```python
from build123d import *

# Parameters (mm, degrees)
BOSS_EXTRUDE1_DEPTH = 457.2
FILLET1_R           = 152.4


with BuildPart() as part:
    # Sketch1 → Boss-Extrude1 (new body)
    with BuildSketch(Plane(origin=(0, 0, 0), x_dir=(0, 0, -1), z_dir=(1, 0, 0))):
        with BuildLine():
            Line((711.548200753, -160.15002575), (669.063267675, -98.166541557))
            Line((669.063267675, -98.166541557), (-541.133997798, 73.322803393))
            Line((-541.133997798, 73.322803393), (-553.825031188, -16.23759413))
            Line((-553.825031188, -16.23759413), (-581.492567074, -11.395775351))
            Line((-581.492567074, -11.395775351), (-581.492567074, 28.611066701))
            Line((-581.492567074, 28.611066701), (-693.769833475, 31.192153284))
            Line((-693.769833475, 31.192153284), (-711.548200753, -33.910775567))
            Line((-711.548200753, -33.910775567), (-671.038221505, -241.199727441))
            Line((-671.038221505, -241.199727441), (-601.675855782, -250.529122735))
            add(Edge.make_bspline(
                [(-601.675855782, -250.529122735), (-541.133997798, -117.43304901), (-401.043539171, -75.545762029)],
                knots=[0, 0, 0, 1, 1, 1], degree=2, weights=[1, 2.246019703, 1]))
            Line((-401.043539171, -75.545762029), (-324.808759835, -85.222901727))
            Line((-324.808759835, -85.222901727), (-338.797926094, -195.427056695))
            Line((-338.797926094, -195.427056695), (-67.759534981, -212.336640741))
            Line((-67.759534981, -212.336640741), (412.240396354, -324.981912238))
            Line((412.240396354, -324.981912238), (412.240396354, -738.576379205))
            add(Edge.make_bspline(
                [(412.240396354, -738.576379205), (426.282298959, -832.127735112), (495.591928337, -872.720699723)],
                knots=[0, 0, 0, 1, 1, 1], degree=2, weights=[1, 2.18722751, 1]))
            Line((495.591928337, -872.720699723), (495.591928337, -904.174333001))
            Line((495.591928337, -904.174333001), (568.451677177, -906.798188592))
            Line((568.451677177, -906.798188592), (669.726727221, -794.275861448))
            Line((669.726727221, -794.275861448), (638.979909752, -220.499963189))
            Line((638.979909752, -220.499963189), (700.473544691, -234.202580835))
            Line((700.473544691, -234.202580835), (711.548200753, -160.15002575))
        make_face()
    extrude(amount=BOSS_EXTRUDE1_DEPTH)

    # Fillet1
    fillet1_edges = [part.edges().sort_by_distance(p)[0] for p in [
        (0, -137.555251504, 691.293211129),
        (0, -1.359311141, 702.659017114),
        (457.2, -137.555251504, 691.293211129),
        (457.2, -1.359311141, 702.659017114),
    ]]
    fillet(fillet1_edges, radius=FILLET1_R)


solid = part.part
```
Model file for the job. Use its own axes, mm. A direction names the side the tool comes from. Coordinates: 2 decimals unless noted, no trailing zeros. Loops run counter-clockwise (first coordinate to the right, second up) from the corner with the lowest first, then second, coordinate; pieces in that order, holes last. Notation, with made-up numbers: (85, 53) - (123, 53) arc R15 ccw to (123, 63) - close; hole circle Ø9 at (-32.75, 51.25). An arc over 180 degrees is marked (long way). Write item = value, one per line. Start each with the question number.
Item 1: Pull direction Z, two halves, no side cores. Call faces 6 (the face through (225.4, -267.87, -168.88)), 7 (the face through (411.372, -141.847, 646.174)), 8 (the face through (225.4, 29.17, 547.39)), 9 (the face through (457.2, -271, -263)): +Z half, -Z half, draft (parallel to the pull), parting line (faces both ways), or undercut.
Item 2: Drop flat-ended pins along their axis: pin 1 Ø4 at (x, y) = (98.5, -148.5) entering from -Z; pin 2 Ø4 at (x, z) = (387.5, -81) entering from +Y; pin 3 Ø1 at (x, y) = (271.5, -53.5) entering from +Z. Give the stop position or say it passes through.
Item 3: Saw through at A-A, the plane z = -31. List the corners of the cut face in (x, y).
Item 4: 3-axis set-ups, long thin cutter, end or side, ignore diameter. For faces 1 (the face through (225.4, -227.255, -669.296)), 2 (the face through (225.4, -203.763, 205.176)), 3 (the face through (225, -888, -495.592)), 4 (the face through (225, 8, 581.493)), 5 (the face through (45.828, -141.847, 646.174)): which of +Z, -Z, +X, -X, +Y, -Y reach the whole face in a straight line?
Item 5: Saw through at B-B, the plane y = -633.5. List the corners of the cut face in (x, z).
Item 6: Wall check: probe 1 along Z at (x, y) = (48.5, -121); probe 2 along Z at (x, y) = (262, -859); probe 3 along Y at (x, z) = (67.5, 171). Give the ranges that are in metal, low to high. Write a range as [from, to].
Answers:
q1.face_6 = undercut
q1.face_7 = +Z half
q1.face_8 = undercut
q1.face_9 = draft
q2.pin_1 = -704.93
q2.pin_2 = -14.55
q2.pin_3 = 707.82
q3.outline = (0, -235.51) - (457.2, -235.51) - (457.2, -7.75) - (0, -7.75) - close
q4.face_1 = +X, -X
q4.face_2 = +X, -X, -Y
q4.face_3 = +Z, +X, -X, -Y
q4.face_4 = +X, -X, +Y
q4.face_5 = +Z, -X, -Y
q5.outline = (0, -661.11) - (457.2, -661.11) - (457.2, -412.24) - (0, -412.24) - close
q6.probe_1 = [-684.71, 329.35], [515.16, 652.85]
q6.probe_2 = [-611.47, -473.26]
q6.probe_3 = [-205.9, 20.87]
